Source: CAD feature listing. Evaluate the final solid. Frame: model axes, mm. A direction names the side the tool comes from. Round coordinates to 2 decimals unless told otherwise and drop trailing zeros. Loops run counter-clockwise (first coordinate to the right, second up) from the corner with the lowest first, then second, coordinate; pieces in that order, holes last.
Item 1: First-contact query: P1, Ø3.5, axis at x = -16.764, y = -32.004, coming from the -Z side. Flat tip, straight axial feed; report the tip coordinate or a pass-through.
Item 2: Ray query, L1, parallel to Y at x = 16.5, z = 4.25; L2, parallel to Y at x = 16, z = 1.25; L3, parallel to X at y = 34, z = 4.25. Return the intervals inside material, ascending.
Item 3: Section query B-B on x = -8.5. Return loops of the section in (y, z), then the cut area to 3 significant figures.
Item 4: Section query C-C on z = 2. Return loops of the section in (x, y), then the cut area to 3 significant figures.
Item 5: Pull-direction query (Y, two-part tool) for faces 3 (the cylindrical face through (16.27, 29.77, 3.13)), 4 (the flat face through (-1, -67.31, 3)), 5 (the flat face through (25, 1, 0)), 6 (the flat face through (-1, 67.31, 3)); classes: released by +Y, released by -Y, zero draft, split by the parting line, or undercut.
Item 6: Section query A-A on y = -9.5. Return loops of the section in (x, z), then the cut area to 3 significant figures.
Item 7: Access query for faces 1 (the flat face through (-20.32, 0, 3)), 2 (the flat face through (25, 1, 6.35)). Directions: +Z, -Z, +X, -X, +Y, -Y. A direction counts if a zero-diameter tool reaches every point of the face in a straight line with its end or side. Return the directions, or none.
```python
from build123d import *

# Parameters (mm, degrees)
F0_W     = 76.2
F0_H     = 134.62
F0_R     = 2.286
F1_DEPTH = 6.35


with BuildPart() as f1:
    # F0 (on Top) → F1 (new body)
    with BuildSketch(Plane.XY):
        Rectangle(F0_W, F0_H)
        Polygon((0, 35.56), (20.32, 35.56), (20.32, 15.24), (20.32, -15.24), (20.32, -35.56), (0, -35.56), (-20.32, -35.56), (-20.32, -15.24), (-20.32, 15.24), (-20.32, 35.56), align=None, mode=Mode.SUBTRACT)
        with BuildLine():
            ThreePointArc((0, -35.56), (-14.36841, -29.60841), (-20.32, -15.24))
            Line((-20.32, -15.24), (-20.32, -35.56))
            Line((-20.32, -35.56), (0, -35.56))
        make_face()
        with Locations((-16.764, -32.004)):
            Circle(F0_R, mode=Mode.SUBTRACT)
        with BuildLine():
            Line((20.32, -35.56), (20.32, -15.24))
            ThreePointArc((20.32, -15.24), (14.36841, -29.60841), (0, -35.56))
            Line((0, -35.56), (20.32, -35.56))
        make_face()
        with Locations((16.764, -32.004)):
            Circle(F0_R, mode=Mode.SUBTRACT)
        with BuildLine():
            ThreePointArc((-20.32, 15.24), (-14.36841, 29.60841), (0, 35.56))
            Line((0, 35.56), (-20.32, 35.56))
            Line((-20.32, 35.56), (-20.32, 15.24))
        make_face()
        with Locations((-16.764, 32.004)):
            Circle(F0_R, mode=Mode.SUBTRACT)
        with BuildLine():
            Line((20.32, 15.24), (20.32, 35.56))
            Line((20.32, 35.56), (0, 35.56))
            ThreePointArc((0, 35.56), (14.36841, 29.60841), (20.32, 15.24))
        make_face()
        with Locations((16.764, 32.004)):
            Circle(F0_R, mode=Mode.SUBTRACT)
    extrude(amount=F1_DEPTH)


solid = f1.part
```
Data:
1. P1: passes through
2. L1: y = -67.31 to -34.27, -29.73 to -27.1, 27.1 to 29.73, 34.27 to 67.31
2. L2: y = -67.31 to -34.16, -29.85 to -27.77, 27.77 to 29.85, 34.16 to 67.31
2. L3: x = -38.1 to -17.88, -15.65 to -7.81, 7.81 to 15.65, 17.88 to 38.1
3. outline: (-67.31, 0) - (-33.7, 0) - (-33.7, 6.35) - (-67.31, 6.35) - close; (33.7, 0) - (67.31, 0) - (67.31, 6.35) - (33.7, 6.35) - close
3. area: 427 mm2
4. outline: (-38.1, -67.31) - (38.1, -67.31) - (38.1, 67.31) - (-38.1, 67.31) - close; hole (-20.32, -15.24) arc R20.32 ccw to (0, -35.56) arc R20.32 ccw to (20.32, -15.24) - (20.32, 15.24) arc R20.32 ccw to (0, 35.56) arc R20.32 ccw to (-20.32, 15.24) - close; hole circle Ø4.57 at (-16.76, -32); hole circle Ø4.57 at (-16.76, 32); hole circle Ø4.57 at (16.76, -32); hole circle Ø4.57 at (16.76, 32)
4. area: 7,660 mm2
5. face 3: undercut
5. face 4: released by -Y
5. face 5: zero draft
5. face 6: released by +Y
6. outline: (-38.1, 0) - (-20.32, 0) - (-20.32, 6.35) - (-38.1, 6.35) - close; (20.32, 0) - (38.1, 0) - (38.1, 6.35) - (20.32, 6.35) - close
6. area: 226 mm2
7. face 1: +Z, -Z
7. face 2: +Z, +X, -X, +Y, -Y
